Autodesk Inventor part; units mm, degrees
ref_plane "YZ Plane" through (0, 0, 0) normal (1, 0, 0) x (0, 1, 0)
ref_plane "XZ Plane" through (0, 0, 0) normal (0, 1, 0) x (-1, 0, 0)
ref_plane "XY Plane" through (0, 0, 0) normal (0, 0, 1) x (1, 0, 0)
sketch "Sketch1" plane through (0, 0, 0) normal (0, 1, 0) x (-1, 0, 0)
  line L0 (0, 0) -> (0, -288.984) construction
  line L1 (5, 0) -> (5, -288.984)
  line L2 (-5, -288.984) -> (-5, 0)
  arc A0 (5, 0) -> (-5, 0) centre (0, 0) ccw
  arc A1 (-5, -288.984) -> (5, -288.984) centre (0, -288.984) ccw
  circle A2 centre (0, 0) radius 1.65
  circle A3 centre (0, -288.984) radius 1.65
  circle A4 centre (0, -231.585) radius 1.65
  arc A5 (-5, -231.585) -> (-5, 0) centre (-593.7207, -115.7925) ccw
  arc A6 (5, -231.585) -> (5, 0) centre (-583.7207, -115.7925) ccw
  point P0 (0, -144.492)
  dimension "d0" = 3.3
  dimension "d1" = 3.3
  dimension "d2" = 10
  dimension "d3" = 288.984
  dimension "d14" = 3.3
  dimension "d15" = 231.585
  dimension "d18" = 600
  dimension "d19" = 600
extrude "Extrusion1" add sketch "Sketch1" along normal blind 6 contours L1 A1 L2 A5 | L1 A5 A6 | L1 A5 A0
Can you work these out from the model? Positions are in its coordinate system, mm. A direction names the side the tool comes from. Coordinates: 2 decimals unless noted, no trailing zeros. Order: outer loops, then holes, each group sorted by start corner. A loop starts at its lowest first (then second) coordinate and runs counter-clockwise, first axis right, second up. Notation, with made-up numbers: (66.5, 79.5) - (97.5, 79.5) arc R20 ccw to (97.5, 102.5) - close; hole circle Ø5 at (-14, -24). An arc over 180 degrees is marked (long way). Answer as a JSON object with one key per item and string values. Group by question number.
Q1. Imagine slicing it at A-A (y = 1.35). Give the number of separate pieces and of enclosed holes in the cut face, and give its area (3 significant figures).
Q2. Imagine slicing it at C-C (z = -62). Please give me the cut outline in (x, y), and give its area (3 significant figures).
Q3. I need wall thicknesses on line 1 (X direction, y = 4.5, z = -245); line 2 (X direction, y = 1.35, z = -121.5). Which ranges of each line are inside material? Lowest first, please. Write a range as from..to.
Q4. On a 3-axis mill with a long thin cutter (end or side, diameter ignored), from which of +Z, -Z, +X, -X, +Y, -Y can I reach the whole of each face in a straight line? I mean faces 1 (the face through (5, 3, -261)), 2 (the face through (-5, 3, -260)). Say none if no direction works.
Q5. Will these pins go through, and if not, where does the flat tip stop? P1, Ø5, axis at x = -5.5, z = -135.5, coming from the -Y side; P2, Ø2, axis at y = 1, z = -152.5, coming from the +X side; P3, Ø3, axis at y = 3.5, z = -184, coming from the -X side; P4, Ø3, axis at y = 3.5, z = -254, coming from the -X side.
Q6. We'd pull the mould along Z, two halves only. Please class faces 3 (the face through (-6.277, 2.958, -114.161)), 4 (the face through (-8, 6, -142)), 5 (the face through (0, 3, 5)), 6 (the face through (-0.11, 2.958, -293.983)): +Z half, -Z half, draft (parallel to the pull), parting line (faces both ways), or undercut.
Determined:
{
 "1": {"separate pieces": "1", "enclosed holes": "3", "area": "2,940 mm2"},
 "2": {"outline": "(-13.86, 0) - (-3.86, 0) - (-3.86, 6) - (-13.86, 6) - close", "area": "60.0 mm2"},
 "3": {"line 1": "x = -5..5", "line 2": "x = -16.25..-6.25"},
 "4": {"face 1": "+Z, -Z, +X, +Y, -Y", "face 2": "-Z, -X, +Y, -Y"},
 "5": {"P1": "stops at y = 0", "P2": "stops at x = -5.09", "P3": "stops at x = -12.56", "P4": "stops at x = -5"},
 "6": {"face 3": "undercut", "face 4": "draft", "face 5": "+Z half", "face 6": "-Z half"}
}
